Design review of the part built by this model. Coordinates are the model's own, in mm. Coordinates: 2 decimals unless noted, no trailing zeros. Write each loop counter-clockwise with the first axis right and the second up, starting at its lowest first coordinate (ties: lowest second). Pieces come first, ordered by that corner, then holes. Notation, with made-up numbers: (37.25, -40) -> (44.25, -40) arc R12 cw to (44.25, -28) -> close; hole circle Ø3 at (58.5, -7). An arc over 180 degrees is marked (long way). Return JSON: item names as keys, results as strings. Group by question number.
from build123d import *

# Parameters (mm, degrees)
F1_DEPTH  = 6.0198
F2_R      = 2.54
F4_DEPTH  = 5.08
F5_W      = 3.8608
F5_H      = 0.889
F5_W_2    = 0.889
F5_H_2    = 3.8608
F6_DEPTH  = 0.3556
F7_W      = 0.889
F7_H      = 0.3556
F7_W_2    = 0.3556
F7_H_2    = 0.889
F8_DEPTH  = 5.08
F9_W      = 1.143
F9_H      = 111.379
F9_W_2    = 65.1002
F9_H_2    = 1.143
F9_W_3    = 72.772369
F10_DEPTH = 1.4224
F11_R     = 0.508


with BuildPart() as f1:
    # F0 (on Top) → F1 (new body)
    with BuildSketch(Plane.XY):
        Polygon((42.2783, 63.5), (-42.2783, 63.5), (-42.2783, -56.642), (-35.4203, -63.5), (35.4203, -63.5), (42.2783, -56.642), align=None)
    extrude(amount=F1_DEPTH)

    # F2
    f2_edges = [f1.edges().sort_by_distance(p)[0] for p in [
        (-42.2783, 63.5, 3.0099),
        (42.2783, 63.5, 3.0099),
    ]]
    fillet(f2_edges, radius=F2_R)

    # F3 (on face) → F4 (cut)
    with BuildSketch(Plane(origin=(0, 0, 0), x_dir=(1, 0, 0), z_dir=(0, 0, -1))):
        Polygon((-39.7383, 55.589898), (-39.7383, -60.96), (39.7383, -60.96), (39.7383, 55.589898), (34.368198, 60.96), (-34.368198, 60.96), align=None)
    extrude(amount=-F4_DEPTH, mode=Mode.SUBTRACT)

    # F5 (on face) → F6 (join)
    with BuildSketch(Plane(origin=(0, 0, 5.08), x_dir=(1, 0, 0), z_dir=(0, 0, -1))):
        with Locations((37.8079, 46.7995)):
            Rectangle(F5_W, F5_H)
        with Locations((37.8079, -0.734602)):
            Rectangle(F5_W, F5_H)
        with Locations((37.8079, -46.7995)):
            Rectangle(F5_W, F5_H)
        with Locations((25.5778, -59.0296)):
            Rectangle(F5_W_2, F5_H_2)
        with Locations((-25.5778, -59.0296)):
            Rectangle(F5_W_2, F5_H_2)
        with Locations((-37.8079, -46.7995)):
            Rectangle(F5_W, F5_H)
        with Locations((-37.8079, -0.734602)):
            Rectangle(F5_W, F5_H)
        with Locations((-37.8079, 46.7995)):
            Rectangle(F5_W, F5_H)
        with Locations((-25.5778, 59.0296)):
            Rectangle(F5_W_2, F5_H_2)
        with Locations((25.5778, 59.0296)):
            Rectangle(F5_W_2, F5_H_2)
    extrude(amount=F6_DEPTH)

    # F7 (on face) → F8 (join)
    with BuildSketch(Plane(origin=(0, 0, 5.08), x_dir=(1, 0, 0), z_dir=(0, 0, -1))):
        with Locations((-25.5778, 60.7822)):
            Rectangle(F7_W, F7_H)
        with Locations((25.5778, 60.7822)):
            Rectangle(F7_W, F7_H)
        with Locations((39.5605, 46.7995)):
            Rectangle(F7_W_2, F7_H_2)
        with Locations((39.5605, -0.734602)):
            Rectangle(F7_W_2, F7_H_2)
        with Locations((-39.5605, 46.7995)):
            Rectangle(F7_W_2, F7_H_2)
        with Locations((-39.5605, -0.734602)):
            Rectangle(F7_W_2, F7_H_2)
        with Locations((-39.5605, -46.7995)):
            Rectangle(F7_W_2, F7_H_2)
        with Locations((-25.5778, -60.7822)):
            Rectangle(F7_W, F7_H)
        with Locations((25.5778, -60.7822)):
            Rectangle(F7_W, F7_H)
        with Locations((39.5605, -46.7995)):
            Rectangle(F7_W_2, F7_H_2)
    extrude(amount=F8_DEPTH)

    # F9 (on face) → F10 (join)
    with BuildSketch(Plane.XY.offset(6.0198)):
        with Locations((-40.4368, 1.9177)):
            Rectangle(F9_W, F9_H)
        with Locations((0, -61.6585)):
            Rectangle(F9_W_2, F9_H_2)
        with Locations((40.4368, 1.9177)):
            Rectangle(F9_W, F9_H)
        with Locations((0.000684, 61.6585)):
            Rectangle(F9_W_3, F9_H_2)
    extrude(amount=F10_DEPTH)

    # F11
    f11_edges = [f1.edges().sort_by_distance(p)[0] for p in [
        (-41.0083, 1.9177, 7.4422),
        (-39.8653, 1.9177, 7.4422),
        (0.000684, 61.087, 7.4422),
        (0.000684, 62.23, 7.4422),
        (39.8653, 1.9177, 7.4422),
        (41.0083, 1.9177, 7.4422),
        (0, -61.087, 7.4422),
        (0, -62.23, 7.4422),
    ]]
    fillet(f11_edges, radius=F11_R)


solid = f1.part
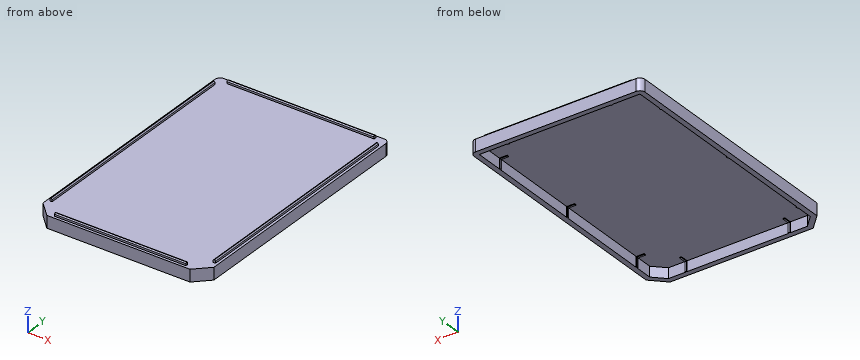
Q1. We need section A-A on x = 9.5. Write out the cut boundary in (y, z) (3 decimals).
Q2. We need section B-B on y = -30. Write out the cut boundary in (x, z), plus the area to 3 significant figures.
Q3. For P1, Ø1, axis at x = 25.5, y = -58.5, coming from the -Z side; P2, Ø0.9, axis at x = -40.5, z = 6.5, coming from the +Y side; P3, Ø4, axis at x = -25.5, y = -3, coming from the +Z side, all flat-tipped, find the tip position at first contact; note any pin that passes through.
Q4. Wall thickness on L1, parallel to Y at x = 26.5, z = 3; L2, parallel to X at y = 30.5, z = 1; L3, parallel to X at y = -29.5, z = 6.25: over which ranges is each line inside the solid? List them lowest first.
Findings below:
{
 "1": {"outline": "(-63.5, 0) -> (-60.96, 0) -> (-60.96, 5.08) -> (60.96, 5.08) -> (60.96, 0) -> (63.5, 0) -> (63.5, 6.02) -> (62.23, 6.02) -> (62.23, 6.934) arc R0.508 ccw to (61.722, 7.442) -> (61.595, 7.442) arc R0.508 ccw to (61.087, 6.934) -> (61.087, 6.02) -> (-61.087, 6.02) -> (-61.087, 6.934) arc R0.508 ccw to (-61.595, 7.442) -> (-61.722, 7.442) arc R0.508 ccw to (-62.23, 6.934) -> (-62.23, 6.02) -> (-63.5, 6.02) -> close"},
 "2": {"outline": "(-42.28, 0) -> (-39.74, 0) -> (-39.74, 5.08) -> (39.74, 5.08) -> (39.74, 0) -> (42.28, 0) -> (42.28, 6.02) -> (41.01, 6.02) -> (41.01, 6.93) arc R0.51 ccw to (40.5, 7.44) -> (40.37, 7.44) arc R0.51 ccw to (39.87, 6.93) -> (39.87, 6.02) -> (-39.87, 6.02) -> (-39.87, 6.93) arc R0.51 ccw to (-40.37, 7.44) -> (-40.5, 7.44) arc R0.51 ccw to (-41.01, 6.93) -> (-41.01, 6.02) -> (-42.28, 6.02) -> close", "area": "108 mm^2"},
 "3": {"P1": "stops at z = 4.72", "P2": "stops at y = 57.61", "P3": "stops at z = 6.02"},
 "4": {"L1": "y = -63.5 to -60.96, 60.96 to 63.5", "L2": "x = -42.28 to -39.74, 39.74 to 42.28", "L3": "x = -41.01 to -39.87, 39.87 to 41.01"}
}
